from build123d import *

# Parameters (mm, degrees)
SKETCH1_W           = 100
SKETCH1_H           = 105
BOSS_EXTRUDE1_DEPTH = 350
SKETCH2_W           = 100
SKETCH2_H           = 105
BOSS_EXTRUDE2_DEPTH = 100
CUT_EXTRUDE1_REACH  = 466.785
SHELL1_T            = -5
CUT_EXTRUDE2_REACH  = 376.584
SKETCH4_R           = 7
CUT_EXTRUDE3_REACH  = 465.957
SKETCH5_W           = 70
SKETCH5_H           = 16
FILLET1_R           = 8


with BuildPart() as part:
    # Sketch1 → Boss-Extrude1 (new body)
    with BuildSketch(Plane(origin=(0, 0, 0), x_dir=(1, 0, 0), z_dir=(0, 1, 0))):
        Rectangle(SKETCH1_W, SKETCH1_H)
    extrude(amount=BOSS_EXTRUDE1_DEPTH)

    # Sketch2 → Boss-Extrude2 (add)
    with BuildSketch(Plane(origin=(0, 350, 0), x_dir=(1, 0, 0), z_dir=(0, 1, 0))):
        Rectangle(SKETCH2_W, SKETCH2_H)
    extrude(amount=BOSS_EXTRUDE2_DEPTH)

    # Sketch3 → Cut-Extrude1 (cut, up to next)
    with BuildSketch(Plane.XY.offset(52.5), mode=Mode.PRIVATE) as cut_extrude1_sk1:
        Polygon((-50, 450), (50, 450), (-50, 379.979246179), align=None)
    cut_extrude1_tool1 = extrude(cut_extrude1_sk1.sketch, amount=-CUT_EXTRUDE1_REACH, mode=Mode.PRIVATE) & part.part
    add(cut_extrude1_tool1.solids().sort_by_distance((-16.666667, 426.659749, 52.5))[0], mode=Mode.SUBTRACT)

    # Shell1
    shell1_openings = [part.faces().sort_by_distance(p)[0] for p in [
        (0, 0, 0),
    ]]
    offset(amount=SHELL1_T, openings=shell1_openings, kind=Kind.INTERSECTION)

    # Sketch4 → Cut-Extrude2 (cut, up to next)
    with BuildSketch(Plane(origin=(-194.98134326, 278.462216729, 0), x_dir=(0.8191520442889949, 0.5735764363510417, 0), z_dir=(-0.5735764363510417, 0.819152044288995, 0)), mode=Mode.PRIVATE) as cut_extrude2_sk1:
        with Locations(Location((251.028269134, 0, 0), (0, 0, 180))):
            Circle(SKETCH4_R)
    cut_extrude2_tool1 = extrude(cut_extrude2_sk1.sketch, amount=-CUT_EXTRUDE2_REACH, mode=Mode.PRIVATE) & part.part
    # Sketch4 → Cut-Extrude2 (cut, up to next)
    with BuildSketch(Plane(origin=(-194.98134326, 278.462216729, 0), x_dir=(0.8191520442889949, 0.5735764363510417, 0), z_dir=(-0.5735764363510417, 0.819152044288995, 0)), mode=Mode.PRIVATE) as cut_extrude2_sk2:
        with Locations(Location((231.528269134, -11.258330249, 0), (0, 0, 180))):
            Circle(SKETCH4_R)
    cut_extrude2_tool2 = extrude(cut_extrude2_sk2.sketch, amount=-CUT_EXTRUDE2_REACH, mode=Mode.PRIVATE) & part.part
    # Sketch4 → Cut-Extrude2 (cut, up to next)
    with BuildSketch(Plane(origin=(-194.98134326, 278.462216729, 0), x_dir=(0.8191520442889949, 0.5735764363510417, 0), z_dir=(-0.5735764363510417, 0.819152044288995, 0)), mode=Mode.PRIVATE) as cut_extrude2_sk3:
        with Locations(Location((231.528269134, 11.258330249, 0), (0, 0, 180))):
            Circle(SKETCH4_R)
    cut_extrude2_tool3 = extrude(cut_extrude2_sk3.sketch, amount=-CUT_EXTRUDE2_REACH, mode=Mode.PRIVATE) & part.part
    add(cut_extrude2_tool1.solids().sort_by_distance((10.648977, 422.446117, 0))[0], mode=Mode.SUBTRACT)
    add(cut_extrude2_tool2.solids().sort_by_distance((-5.324488, 411.261376, 11.25833))[0], mode=Mode.SUBTRACT)
    add(cut_extrude2_tool3.solids().sort_by_distance((-5.324488, 411.261376, -11.25833))[0], mode=Mode.SUBTRACT)

    # Sketch5 → Cut-Extrude3 (cut, up to next)
    with BuildSketch(Plane.ZY.offset(50), mode=Mode.PRIVATE) as cut_extrude3_sk1:
        with Locations((0, 361.979246179)):
            Rectangle(SKETCH5_W, SKETCH5_H)
    cut_extrude3_tool1 = extrude(cut_extrude3_sk1.sketch, amount=-CUT_EXTRUDE3_REACH, mode=Mode.PRIVATE) & part.part
    add(cut_extrude3_tool1.solids().sort_by_distance((-50, 361.979246, 0))[0], mode=Mode.SUBTRACT)

    # Fillet1
    fillet1_edges = [part.edges().sort_by_distance(p)[0] for p in [
        (-47.5, 353.979246179, 35),
        (-47.5, 369.979246179, 35),
        (-47.5, 353.979246179, -35),
        (-47.5, 369.979246179, -35),
    ]]
    fillet(fillet1_edges, radius=FILLET1_R - 0.0001)  # a hair under: the kernel refuses the full size


solid = part.part
Can you work these out from the model? Positions are in its coordinate system, mm. A direction names the side the tool comes from. Coordinates: 2 decimals unless noted, no trailing zeros. Write each loop counter-clockwise with the first axis right and the second up, starting at its lowest first coordinate (ties: lowest second). Pieces come first, ordered by that corner, then holes.
Q1. Imagine slicing it at A-A, the plane y = 94. List the corners of the cut face in (x, z) for me, plus the area to 3 significant figures.
Results found:
outline: (-50, -52.5) - (50, -52.5) - (50, 52.5) - (-50, 52.5) - close; hole (-45, -47.5) - (45, -47.5) - (45, 47.5) - (-45, 47.5) - close
area: 1,950 mm2
Q2. Please list where these lines run through material, in increasing order: L1, parallel to Z at x = 7, y = 230; L2, parallel to X at y = 342.5, z = -37.5; L3, parallel to X at y = 387, z = -14.
Results found:
L1: z = -52.5 to -47.5, 47.5 to 52.5
L2: x = -50 to -45, 45 to 50
L3: x = -39.97 to -31.26, 45 to 50
Q3. Which directions (+Z, -Z, +X, -X, +Y, -Y) give clear straight access to the entire face, cutting with the end or side of a thin tool? Please do faces 4 (the face through (-48, 0, 0)), 5 (the face through (-1, 217, 47.5)), 6 (the face through (-47.46, 367.7, -32.59)).
Results found:
face 4: +Z, -Z, +X, -X, -Y
face 5: -Y
face 6: -X
Q4. Imagine slicing it at B-B, the plane x = 41. List the corners of the cut face in (y, z) for me, plus the area to 3 significant figures.
Results found:
outline: (0, -52.5) - (443.7, -52.5) - (443.7, 52.5) - (0, 52.5) - (0, 47.5) - (437.59, 47.5) - (437.59, -47.5) - (0, -47.5) - close
area: 5,020 mm2
Q5. For P1, Ø1, axis at x = 18.5, z = -12.5, coming from the +Y side; P2, Ø2.5, axis at x = -46.5, z = 11, coming from the +Y side; P3, Ø1.5, axis at x = 10, z = 28.5, coming from the +Y side, each with a flat end and sliding along its axis, tell me the tip position at first contact or that it passes through.
Results found:
P1: stops at y = 428.29
P2: stops at y = 383.31
P3: stops at y = 422.52
Q6. If we mould it in two halves opening along X, with no side actions, what happens to faces 1 (the face through (-1, 222, -52.5)), 2 (the face through (-50, 187, 1)), 3 (the face through (-9.38, 405.41, 13.36))? For each: +X half, -X half, draft (parallel to the pull), parting line (faces both ways), or undercut.
Results found:
face 1: draft
face 2: -X half
face 3: undercut
Q7. Imagine slicing it at C-C, the plane x = -2.5. Count the separate pieces of the cut face and the enclosed holes in it, plus the area to 3 significant figures.
Results found:
separate pieces: 3
enclosed holes: 0
area: 4,550 mm2
